```python
from build123d import *

# Parameters (mm, degrees)
F0_R     = 10
F1_DEPTH = 25
F3_R     = 100
F4_DEPTH = 132
F5_R     = 53.5394433614
F6_DEPTH = 50


with BuildPart() as f1:
    # F0 (on Top) → F1 (new body)
    with BuildSketch(Plane.XY):
        Circle(F0_R)
    extrude(amount=F1_DEPTH)


with BuildPart() as f4:
    # F3 (on Top) → F4 (new body)
    with BuildSketch(Plane.XY):
        Circle(F3_R)
    extrude(amount=F4_DEPTH)

    # F5 (on face) → F6 (cut)
    with BuildSketch(Plane.XY.offset(132)):
        Circle(F5_R)
    extrude(amount=-F6_DEPTH, mode=Mode.SUBTRACT)


solid = f4.part
```
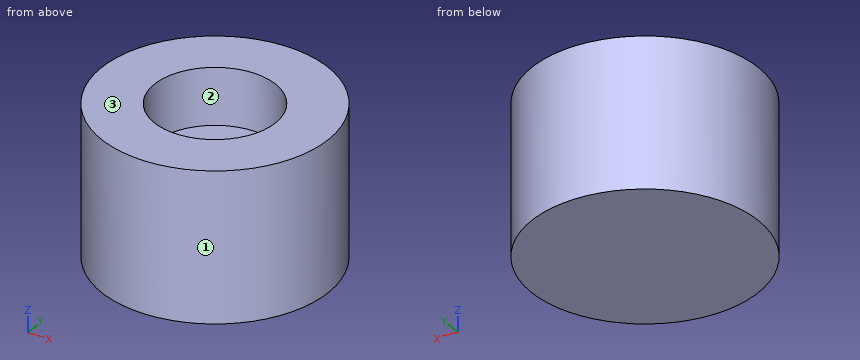
Check sheet for the modelled part. Datum: model origin and axes. Units: mm. Face numbers are marked on the shaded views. Coordinates: 2 decimals unless noted, no trailing zeros. Write each loop counter-clockwise with the first axis right and the second up, starting at its lowest first coordinate (ties: lowest second). Pieces come first, ordered by that corner, then holes. Notation, with made-up numbers: (-24, 62) - (0, 62) arc R29 ccw to (0, 87) - close; hole circle Ø8 at (-33.75, 37). An arc over 180 degrees is marked (long way). One line per question, with ' | ' between items.
Item 1: Thickness scan on line 1 (Y direction, x = 0, z = 116); line 2 (Z direction, x = 36.5, y = -13); line 3 (Y direction, x = -31, z = 95). Record the ranges inside material, lowest first. Write a range as [from, to].
Determined:
line 1: y = [-100, -53.54], [53.54, 100] | line 2: z = [0, 82] | line 3: y = [-95.07, -43.65], [43.65, 95.07]
Item 2: Sectioned sample at D-D on z = 78. Record the boundary of the cut face in (x, y), plus the area to 3 significant figures.
Determined:
outline: circle Ø200 at (0, 0) | area: 31,400 mm2
Item 3: Mould release check, pull along X, two halves, no side actions. Record for the marked faces 1, 2 and 3: pulls with the +X half, pulls with the -X half, needs draft (parallel to the pull), parting line crosses it, or undercut.
Determined:
face 1: parting line crosses it | face 2: undercut | face 3: needs draft
Item 4: Gauge pin test, flat ends, axial feed: P1, Ø10, axis at y = 69, z = 37, coming from the +X side; P2, Ø10, axis at x = 59, z = 100, coming from the +Y side; P3, Ø6, axis at x = 8, z = 93, coming from the +Y side. Record the tip position at first contact, or that the pin passes through.
Determined:
P1: stops at x = 76.84 | P2: stops at y = 84.17 | P3: stops at y = 99.87
Item 5: Sectioned sample at B-B on y = 0. Record the boundary of the cut face in (x, z), plus the area to 3 significant figures.
Determined:
outline: (-100, 0) - (100, 0) - (100, 132) - (53.54, 132) - (53.54, 82) - (-53.54, 82) - (-53.54, 132) - (-100, 132) - close | area: 21,000 mm2
Item 6: Sectioned sample at A-A on z = 121.5. Record the boundary of the cut face in (x, y), plus the area to 3 significant figures.
Determined:
outline: circle Ø200 at (0, 0); hole circle Ø107.08 at (0, 0) | area: 22,400 mm2
